from build123d import *

# Parameters (mm, degrees)
F0_W            = 304.8
F0_H            = 203.2
F1_DEPTH        = 19.05
F2_W            = 228.6
F2_H            = 25.4
F3_DEPTH        = 19.051
F5_D            = 6.35
F6_R            = 6.35
F8_D            = 12.7
F9_R            = 6.35
F10_DEPTH       = 12.7
F12_D           = 9.525
F12_CBORE_D     = 15.875
F12_CBORE_DEPTH = 12.7
F13_SIZE        = 50.8


with BuildPart() as f1:
    # F0 (on Front) → F1 (new body)
    with BuildSketch(Plane.XZ):
        with Locations((152.4, 101.6)):
            Rectangle(F0_W, F0_H)
    extrude(amount=F1_DEPTH)

    # F2 (on face) → F3 (cut, through all)
    with BuildSketch(Plane.XZ.offset(19.05)):
        with Locations((152.4, 12.7)):
            Rectangle(F2_W, F2_H)
    extrude(amount=-F3_DEPTH, mode=Mode.SUBTRACT)

    # F5 (through all)
    with Locations(Plane.XZ.offset(19.05)):
        with Locations((120.65, 38.1), (184.15, 38.1)):
            Hole(F5_D / 2)

    # F6
    f6_edges = [f1.edges().sort_by_distance(p)[0] for p in [
        (38.1, -9.525, 25.4),
        (38.1, -9.525, 0),
        (0, -9.525, 0),
        (266.7, -9.525, 25.4),
        (266.7, -9.525, 0),
        (304.8, -9.525, 0),
    ]]
    fillet(f6_edges, radius=F6_R)

    # F8 (through all)
    with Locations(Plane.XZ.offset(19.05)):
        with Locations((152.4, 105.6132)):
            Hole(F8_D / 2)

    # F9 (on face) → F10 (cut)
    with BuildSketch(Plane(origin=(0, 0, 0), x_dir=(-1, 0, 0), z_dir=(0, 1, 0))):
        with Locations((-25.4, 134.1882)):
            Circle(F9_R)
        with Locations((-279.4, 134.1882)):
            Circle(F9_R)
    extrude(amount=-F10_DEPTH, mode=Mode.SUBTRACT)

    # F12 (through all)
    with Locations(Plane(origin=(0, 0, 0), x_dir=(-1, 0, 0), z_dir=(0, 1, 0))):
        with Locations((-285.75, 95.25), (-285.75, 19.05), (-19.05, 19.05), (-19.05, 95.25)):
            CounterBoreHole(F12_D / 2, F12_CBORE_D / 2, F12_CBORE_DEPTH)

    # F13
    f13_edges = [f1.edges().sort_by_distance(p)[0] for p in [
        (0, -9.525, 203.2),
        (304.8, -9.525, 203.2),
    ]]
    chamfer(f13_edges, length=F13_SIZE)


solid = f1.part
Verification items for the finished model (mm, model axes). A direction names the side the tool comes from. Coordinates: 2 decimals unless noted, no trailing zeros. Write each loop counter-clockwise with the first axis right and the second up, starting at its lowest first coordinate (ties: lowest second). Pieces come first, ordered by that corner, then holes. Notation, with made-up numbers: (74.25, 19.25) - (101.25, 19.25) arc R26 ccw to (101.25, 36.25) - close; hole circle Ø11 at (-30.75, 34.25). An arc over 180 degrees is marked (long way). Answer as a JSON object with one key per item and string values.
(1) Thickness scan on line 1 along Z through (x, y) = (19.05, -17.25); line 2 along Z through (x, y) = (253, -17.25); line 3 along Z through (x, y) = (273, -2). Record the ranges inside material, lowest first.
Report:
{"line 1": "0 to 14.29, 23.81 to 90.49, 100.01 to 171.45", "line 2": "25.4 to 203.2", "line 3": "0 to 184.2"}
(2) Cross-section at A-A on x = 184.15. Record the cut outline in (y, z) (3 decimals), plus the area to 3 significant figures.
Report:
{"outline": "(-19.05, 25.4) - (0, 25.4) - (0, 34.925) - (-19.05, 34.925) - close; (-19.05, 41.275) - (0, 41.275) - (0, 203.2) - (-19.05, 203.2) - close", "area": "3,270 mm^2"}
(3) Tool access check on faces 1 (the cylindrical face through (15.54, -15.92, 22.27)), 2 (the flat face through (151, -10, 25.4)), 3 (the flat face through (14, -12.7, 95)). Record the directions out of +Z, -Z, +X, -X, +Y, -Y that give a thin tool (end or side, any length) a straight path to the whole face; none if there is none.
Report:
{"face 1": "+Y, -Y", "face 2": "-Z, +Y, -Y", "face 3": "+Y"}
(4) Cross-section at B-B on z = 95.25. Record the cut outline in (x, y).
Report:
{"outline": "(0, -19.05) - (14.29, -19.05) - (14.29, -12.7) - (11.11, -12.7) - (11.11, 0) - (0, 0) - close; (23.81, -19.05) - (280.99, -19.05) - (280.99, -12.7) - (277.81, -12.7) - (277.81, 0) - (26.99, 0) - (26.99, -12.7) - (23.81, -12.7) - close; (290.51, -19.05) - (304.8, -19.05) - (304.8, 0) - (293.69, 0) - (293.69, -12.7) - (290.51, -12.7) - close"}
(5) Gauge pin test, flat ends, axial feed: pin 1 Ø4 at (x, z) = (248, 45) entering from +Y; pin 2 Ø5 at (x, z) = (284.5, 18.5) entering from +Y; pin 3 Ø8 at (x, z) = (21.5, 21) entering from +Y; pin 4 Ø9.5 at (x, y) = (161.5, -7) entering from -Z. Record the tip position at first contact, or that the pin passes through.
Report:
{"pin 1": "y = 0", "pin 2": "through", "pin 3": "y = -12.7", "pin 4": "z = 25.4"}
(6) Mould release check, pull along Z, two halves, no side actions. Record for faces 4 (the flat face through (25.8, -9.4, 178.2)), 5 (the cylindrical face through (123.82, -9.39, 38.24)), 6 (the flat face through (0, -9, 78)), 7 (the cylindrical face through (264.79, -9.39, 23.59)): pulls with the +Z half, pulls with the -Z half, needs draft (parallel to the pull), parting line crosses it, or undercut.
Report:
{"face 4": "pulls with the +Z half", "face 5": "undercut", "face 6": "needs draft", "face 7": "pulls with the -Z half"}
(7) Cross-section at C-C on x = 152.4. Record the cut outline in (y, z), plus the area to 3 significant figures.
Report:
{"outline": "(-19.05, 25.4) - (0, 25.4) - (0, 99.26) - (-19.05, 99.26) - close; (-19.05, 111.96) - (0, 111.96) - (0, 203.2) - (-19.05, 203.2) - close", "area": "3,150 mm^2"}
(8) Cross-section at D-D on y = -5.75. Give the number of separate pieces and of enclosed holes in the cut face, plus the area to 3 significant figures.
Report:
{"separate pieces": "1", "enclosed holes": "9", "area": "52,300 mm^2"}
